Autodesk Inventor part; units mm, degrees
ref_plane "YZ Plane" through (0, 0, 0) normal (1, 0, 0) x (0, 1, 0)
ref_plane "XZ Plane" through (0, 0, 0) normal (0, 1, 0) x (-1, 0, 0)
ref_plane "XY Plane" through (0, 0, 0) normal (0, 0, 1) x (1, 0, 0)
sketch "スケッチ1" plane through (0, 0, 0) normal (0, 0, 1) x (1, 0, 0)
  line L0 (-16, -16) -> (16, -16)
  line L1 (16, -16) -> (16, 16)
  line L2 (16, 16) -> (-16, 16)
  line L3 (-16, 16) -> (-16, -16)
  line L4 (-16, -16) -> (16, 16) construction
  line L5 (16, -16) -> (-16, 16) construction
  line L6 (-14.4, 14.4) -> (14.4, 14.4)
  line L7 (14.4, 14.4) -> (14.4, -14.4)
  line L8 (14.4, -14.4) -> (-14.4, -14.4)
  line L9 (-14.4, -14.4) -> (-14.4, 14.4)
  point P0 (0, 0)
  dimension "d0" = 32
  dimension "d1" = 32
  dimension "d2" = 1.6
extrude "押し出し1" add sketch "スケッチ1" along normal blind 45
sketch "スケッチ2" plane through (-16, 16, 0) normal (0, 1, 0) x (1, 0, 0)
  circle A0 centre (16, 0) radius 13.6
  dimension "d5" = 27.2
extrude "押し出し2" cut sketch "スケッチ2" against normal blind 32
sketch "スケッチ3" plane through (-16, 16, 45) normal (0, 1, 0) x (1, 0, 0)
  line L0 (32, 0) -> (0, 0)
  point P0 (16, 45)
  point P1 (16, 15)
  dimension "d16" = 30
hole "穴1" at (0, 16, 30) direction (0, -1, 0) diameter 10.5 end through all
sketch "スケッチ4" plane through (-16, 16, 45) normal (0, 1, 0) x (1, 0, 0)
  circle A0 centre (16, 15) radius 13.6
  point P0 (16, 45)
  dimension "d17" = 30
  dimension "d18" = 27.2
properties part number "軸受上用"
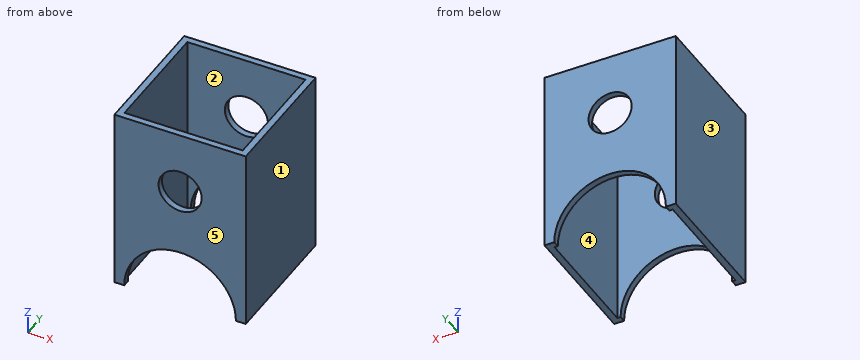
Geometry: final body of the model. Coordinates: model frame, mm. Face numbers are marked on the shaded views. A direction names the side the tool comes from. Coordinates: 2 decimals unless noted, no trailing zeros. Order: outer loops, then holes, each group sorted by start corner. A loop starts at its lowest first (then second) coordinate and runs counter-clockwise, first axis right, second up.
Item 1: Material intervals for line 1 along Y through (x, z) = (10, 28.5); line 2 along Z through (x, y) = (0, -14.9); line 3 along X through (y, z) = (14.8, 30), sorted ascending.
Answer:
line 1: y = -16 to -14.4, 14.4 to 16
line 2: z = 13.6 to 24.75, 35.25 to 45
line 3: x = -16 to -5.25, 5.25 to 16
Item 2: Access query for the marked faces 1 and 2. Directions: +Z, -Z, +X, -X, +Y, -Y. A direction counts if a zero-diameter tool reaches every point of the face in a straight line with its end or side. Return the directions, or none.
Answer:
face 1: +Z, -Z, +X, +Y, -Y
face 2: +Z, -Z
Item 3: Section query A-A (x = 0). Output: boundary loops of the cut face in (y, z).
Answer:
outline: (-16, 13.6) - (-14.4, 13.6) - (-14.4, 24.75) - (-16, 24.75) - close; (-16, 35.25) - (-14.4, 35.25) - (-14.4, 45) - (-16, 45) - close; (14.4, 13.6) - (16, 13.6) - (16, 24.75) - (14.4, 24.75) - close; (14.4, 35.25) - (16, 35.25) - (16, 45) - (14.4, 45) - close
Item 4: Section query D-D (z = 39). Output: boundary loops of the cut face in (x, y), then the cut area to 3 significant figures.
Answer:
outline: (-16, -16) - (16, -16) - (16, 16) - (-16, 16) - close; hole (-14.4, -14.4) - (14.4, -14.4) - (14.4, 14.4) - (-14.4, 14.4) - close
area: 195 mm2
Item 5: Section query B-B (y = 0.5). Output: boundary loops of the cut face in (x, z), then the cut area to 3 significant figures.
Answer:
outline: (-16, 0) - (-14.4, 0) - (-14.4, 45) - (-16, 45) - close; (14.4, 0) - (16, 0) - (16, 45) - (14.4, 45) - close
area: 144 mm2
Item 6: Draft query along Y for the marked faces 3, 4 and 5. Return one class per face: released by +Y, released by -Y, zero draft, split by the parting line, or undercut.
Answer:
face 3: zero draft
face 4: undercut
face 5: released by -Y
Item 7: Section query C-C (z = 30). Output: boundary loops of the cut face in (x, y).
Answer:
outline: (-16, -16) - (-5.25, -16) - (-5.25, -14.4) - (-14.4, -14.4) - (-14.4, 14.4) - (-5.25, 14.4) - (-5.25, 16) - (-16, 16) - close; (5.25, -16) - (16, -16) - (16, 16) - (5.25, 16) - (5.25, 14.4) - (14.4, 14.4) - (14.4, -14.4) - (5.25, -14.4) - close
